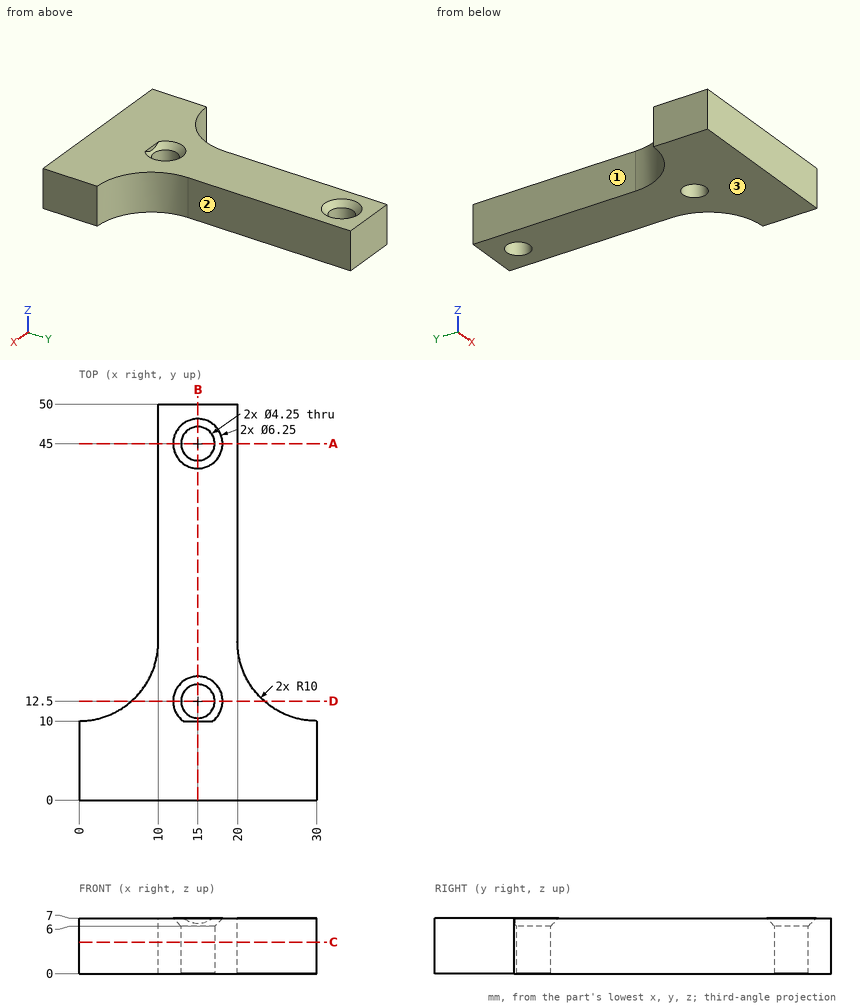
Answer from the drawing. Dimensions are ordinates in mm from the lowest x, y and z of the part. A direction names the side the tool comes from. Coordinates: 2 decimals unless noted, no trailing zeros. Loops run counter-clockwise (first coordinate to the right, second up) from the corner with the lowest first, then second, coordinate; pieces in that order, holes last. Notation, with made-up numbers: (-34, -11.5) -> (-23, -11.5) arc R19 ccw to (-23, 12.5) -> close; hole circle Ø7 at (56, -33). An arc over 180 degrees is marked (long way). Answer in a Markdown table with one row per item.
Item 1: A cutting plane is placed at D-D on y = 12.5. Determine the outline of the cut face in (x, z) (1 decimal).
Returned:
| item | result |
|---|---|
| outline | (6.6, 0) -> (12.9, 0) -> (12.9, 6) -> (11.9, 7) -> (6.6, 7) -> close; (17.1, 0) -> (23.4, 0) -> (23.4, 7) -> (18.1, 7) -> (17.1, 6) -> close |
Item 2: Each of these flat-tipped pins is pushed along its axis until it touches: P1, Ø2, axis at y = 33.5, z = 5, coming from the -X side; P2, Ø3, axis at y = 40, z = 2.5, coming from the +X side. Where does it stop, or does it pass through?
Returned:
| item | result |
|---|---|
| P1 | stops at x = 10 |
| P2 | stops at x = 20 |
Item 3: A cutting plane is placed at A-A on y = 45. Determine the outline of the cut face in (x, z) (3 decimals).
Returned:
| item | result |
|---|---|
| outline | (10, 0) -> (12.875, 0) -> (12.875, 6) -> (11.875, 7) -> (10, 7) -> close; (17.125, 0) -> (20, 0) -> (20, 7) -> (18.125, 7) -> (17.125, 6) -> close |
Item 4: Straight lines are drawn through the part: line 1 along Y through (x, z) = (15, 2.25) (3 decimals); line 2 along Y through (x, z) = (13.5, 1.75) (1 decimal); line 3 along X through (y, z) = (23.5, 6.75). For each, find the intervals that lie inside material, in ascending order. Write a range as [from, to].
Returned:
| item | result |
|---|---|
| line 1 | y = [0, 10.375], [14.625, 42.875], [47.125, 50] |
| line 2 | y = [0, 11], [14, 43.5], [46.5, 50] |
| line 3 | x = [10, 20] |
Item 5: A cutting plane is placed at C-C on z = 4. Give the number of separate pieces and of enclosed holes in the cut face, plus the area to 3 significant figures.
Returned:
| item | result |
|---|---|
| separate pieces | 1 |
| enclosed holes | 2 |
| area | 715 mm^2 |
Item 6: A cutting plane is placed at B-B on x = 15. Determine the outline of the cut face in (y, z) (3 decimals), plus the area to 3 significant figures.
Returned:
| item | result |
|---|---|
| outline | (0, 0) -> (10.375, 0) -> (10.375, 6) -> (10, 6.375) -> (10, 7) -> (0, 7) -> close; (14.625, 0) -> (42.875, 0) -> (42.875, 6) -> (41.875, 7) -> (15.625, 7) -> (14.625, 6) -> close; (47.125, 0) -> (50, 0) -> (50, 7) -> (48.125, 7) -> (47.125, 6) -> close |
| area | 289 mm^2 |
Item 7: For the marked faces 1, 2 and 3, determine the directions among +Z, -Z, +X, -X, +Y, -Y from which every point of the face is accessible in a straight line to the end or side of a thin tool.
Returned:
| item | result |
|---|---|
| face 1 | +Z, -Z, -X, +Y |
| face 2 | +Z, -Z, +X, +Y |
| face 3 | -Z, +X, -X, +Y, -Y |
